from build123d import *

# Parameters (mm, degrees)
F0_W     = 80
F0_H     = 68
F0_R     = 2.75
F1_DEPTH = 3
F3_ANGLE = 180


with BuildPart() as f1:
    # F0 (on Front) → F1 (new body)
    with BuildSketch(Plane.XZ):
        with Locations((-45.665469, 40.798562)):
            Rectangle(F0_W, F0_H)
        with Locations((-10.665469, 40.798562)):
            Circle(F0_R, mode=Mode.SUBTRACT)
    extrude(amount=F1_DEPTH)


with BuildPart() as f3_1:
    # F3: copy of F1
    add(f1.part.rotate(Axis((-5.665469, -1.5, 40.798562), (0, 1, 0)), F3_ANGLE))


solid = f1.part
Geometry: final body of the model. Coordinates: model frame, mm. Give positions to 0.01 mm unless a question says otherwise; leave off trailing zeros. Answer as CSV lines item,"result". Start each with the question number.
1. Ray query, L1, parallel to X at y = -1.45, z = 40; L2, parallel to Z at x = -12, y = -1.9; L3, parallel to Z at x = -10, y = -0.4. Return the intervals inside material, ascending.
2. Draft query along X for faces 1 (the face through (-85.665, -1, 40)), 2 (the face through (-5.665, -1, 40)), 3 (the face through (-8.04, -1.48, 41.62)), 4 (the face through (-46, 0, 41)). Return one class per face: released by +X, released by -X, zero draft, split by the parting line, or undercut.
3. Pin query (flat end, axial travel): P1, Ø2, axis at x = -61.5, z = 48.5, coming from the +Y side. Return the tip coordinate at first contact, or that it passes through.
Answers:
1,L1,"x = -85.67 to -13.3, -8.03 to -5.67"
1,L2,"z = 6.8 to 38.39, 43.2 to 74.8"
1,L3,"z = 6.8 to 38.13, 43.47 to 74.8"
2,face 1,"released by -X"
2,face 2,"released by +X"
2,face 3,"undercut"
2,face 4,"zero draft"
3,P1,"stops at y = 0"
